Check sheet for the drawn part. Datum: minimum x, y, z corner. Units: mm. A direction names the side the tool comes from. Give positions to 0.01 mm unless a question says otherwise; leave off trailing zeros. Write each loop counter-clockwise with the first axis right and the second up, starting at its lowest first coordinate (ties: lowest second). Pieces come first, ordered by that corner, then holes.
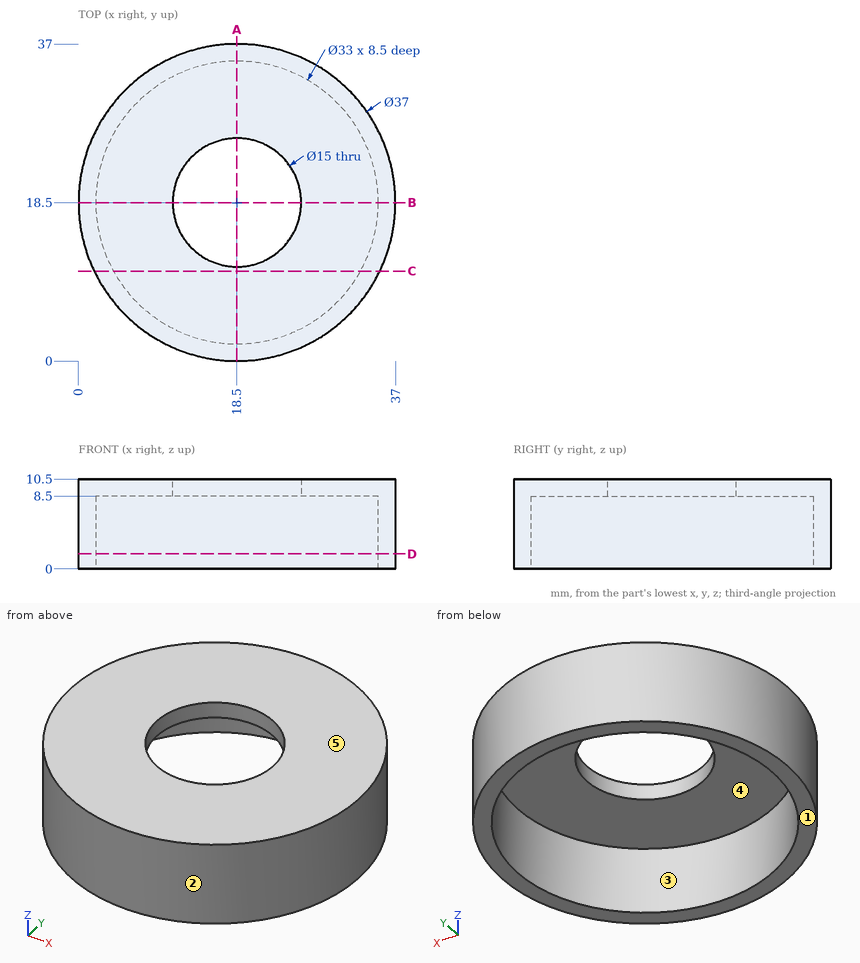
1) Gauge pin test, flat ends, axial feed: pin 1 (5 mm diameter, centred on y = 23, z = 5, fed in from +X); pin 2 (2 mm diameter, centred on y = 24.5, z = 6.5, fed in from -X); pin 3 (10 mm diameter, centred on x = 16.5, y = 13, fed in from -Z). Record the tip position at first contact, or that the pin passes through.
2) Sectioned sample at D-D on z = 1.75. Record the boundary of the cut face in (x, y).
3) Access from +Z, -Z, +X, -X, +Y, -Y to the whole of each face (thin tool, end or side, straight path). Record for the marked faces 4 and 5.
4) Draft check along Y on the marked faces 1, 2 and 3. Enter one of: +Y half, -Y half, draft (parallel to the pull), parting line (faces both ways), or undercut.
5) Scan lines: L1, parallel to Y at x = 18.5, z = 5; L2, parallel to X at y = 13.5, z = 5.5; L3, parallel to X at y = 15, z = 4.75. Record each from-to range of solid material in increasing order.
6) Sectioned sample at A-A on x = 18.5. Record the boundary of the cut face in (y, z).
7) Sectioned sample at C-C on y = 10.5. Record the boundary of the cut face in (x, z).
Answers below:
1. pin 1: stops at x = 36.89
1. pin 2: stops at x = 0.69
1. pin 3: stops at z = 8.5
2. outline: circle Ø37 at (18.5, 18.5); hole circle Ø33 at (18.5, 18.5)
3. face 4: -Z
3. face 5: +Z, +X, -X, +Y, -Y
4. face 1: draft
4. face 2: parting line
4. face 3: undercut
5. L1: y = 0 to 2, 35 to 37
5. L2: x = 0.69 to 2.78, 34.22 to 36.31
5. L3: x = 0.33 to 2.38, 34.62 to 36.67
6. outline: (0, 0) - (2, 0) - (2, 8.5) - (11, 8.5) - (11, 10.5) - (0, 10.5) - close; (26, 8.5) - (35, 8.5) - (35, 0) - (37, 0) - (37, 10.5) - (26, 10.5) - close
7. outline: (1.82, 0) - (4.07, 0) - (4.07, 8.5) - (32.93, 8.5) - (32.93, 0) - (35.18, 0) - (35.18, 10.5) - (1.82, 10.5) - close
